The listing builds one solid part. Answer for the finished solid, in the listing's coordinates (mm). A direction names the side the tool comes from. Round coordinates to 2 decimals unless told otherwise and drop trailing zeros. Write each loop counter-clockwise with the first axis right and the second up, starting at its lowest first coordinate (ties: lowest second). Pieces come first, ordered by that corner, then holes. Notation, with made-up numbers: (36, 18) - (64, 18) arc R11 cw to (64, 24) - close; hole circle Ø7 at (84.25, 47.5). An arc over 180 degrees is marked (long way). Return JSON: item names as keys, results as strings. Group by question number.
(1) Which of the six approach directions +Z, -Z, +X, -X, +Y, -Y give full straight-line access (tool end or side, diameter ignored) to faces 1 (the cylindrical face through (11.331, 39.567, -36.024)), 2 (the cylindrical face through (15.722, 3.565, 0.423))?
(2) Determine the mould class of faces 3 (the cylindrical face through (-6.834, 2.974, -1.517)), 4 (the cylindrical face through (-11.517, 39.567, 35.956)), 5 (the cylindrical face through (-27.16, 39.57, 41.47)), 6 (the flat face through (7, 42.032, 1)) for opening direction Z: +Z half, -Z half, draft (parallel to the pull), parting line (faces both ways), or undercut.
(3) Section A-A, the plane x = -5 is taken. Give the number of separate pieces and of enclosed holes in the cut face, then the cut area to 3 significant figures.
(4) Section C-C, the plane z = 22 is taken. Write down the section's boundary in (x, y).
(5) Find the intervals of material crossed by line 1 along X through (y, z) = (3, 0) (3 decimals); line 2 along Y through (x, z) = (6, 14); line 3 along X through (y, z) = (6.5, 0) (3 decimals), in increasing order. Write a range as [from, to].
(6) Each of these flat-tipped pins is pushed along its axis until it touches: pin 1 (6 mm diameter, centred on x = -15, y = 34, fed in from +Z); pin 2 (3.5 mm diameter, centred on x = -6.096, z = 38.1, fed in from +Y); pin 3 (1 mm diameter, centred on y = 37, z = 30, fed in from -X); pin 4 (17 mm diameter, centred on x = 0, z = 0, fed in from +Y). Where does it stop, or does it pass through?
(7) Section D-D, the plane y = 19.5 is taken. Write down the section's boundary in (x, z) (3 decimals), then the cut area to 3 significant figures.
(8) Section B-B, the plane z = -12.5 is taken. Write down the section's boundary in (x, y).
```python
from build123d import *

# Parameters (mm, degrees)
SKETCH1_R                      = 34.925
SKETCH1_R_2                    = 7
BOSS_EXTRUDE1_DEPTH            = 7.032
SKETCH2_R                      = 7.5
CUT_EXTRUDE1_DEPTH             = 1
BOSS_EXTRUDE2_DEPTH            = 30
CUT_EXTRUDE2_DEPTH             = 58.78850448
SKETCH6_R                      = 34.925
SKETCH6_R_2                    = 6.6
BOSS_EXTRUDE6_DEPTH            = 5
CBORE_FOR_M3_SHCS1_D           = 3.3
CBORE_FOR_M3_SHCS1_DEPTH       = 5
CBORE_FOR_M3_SHCS1_CBORE_D     = 6.5
CBORE_FOR_M3_SHCS1_CBORE_DEPTH = 3
SKETCH9_R                      = 3.25
CUT_EXTRUDE3_DEPTH             = 62.732327625
SKETCH10_R                     = 2.2479
BOSS_EXTRUDE7_DEPTH            = 5


with BuildPart() as part:
    # Sketch1 → Boss-Extrude1 (new body)
    with BuildSketch(Plane(origin=(0, 0, 0), x_dir=(1, 0, 0), z_dir=(0, 1, 0))):
        with Locations(Location((0, 0, 0), (0, 0, 270))):
            Circle(SKETCH1_R)
        with Locations(Location((0, 0, 0), (0, 0, 270))):
            Circle(SKETCH1_R_2, mode=Mode.SUBTRACT)
    extrude(amount=BOSS_EXTRUDE1_DEPTH)

    # Sketch2 → Cut-Extrude1 (cut)
    with BuildSketch(Plane(origin=(0, 7.032, 0), x_dir=(1, 0, 0), z_dir=(0, 1, 0))):
        with Locations(Location((0, 0, 0), (0, 0, 270))):
            Circle(SKETCH2_R)
    extrude(amount=-CUT_EXTRUDE1_DEPTH, mode=Mode.SUBTRACT)

    # Sketch3 → Boss-Extrude2 (add)
    with BuildSketch(Plane(origin=(0, 7.032, 0), x_dir=(1, 0, 0), z_dir=(0, 1, 0))):
        with BuildLine():
            Line((19.05, 25.4), (19.05, 29.272053652))
            ThreePointArc((19.05, 29.272053652), (-34.925, 0), (19.05, -29.272053652))
            Line((19.05, -29.272053652), (19.05, -25.4))
            Line((19.05, -25.4), (13.090860361, -25.4))
            ThreePointArc((13.090860361, -25.4), (-28.575, 0), (13.090860361, 25.4))
            Line((13.090860361, 25.4), (19.05, 25.4))
        make_face()
    extrude(amount=BOSS_EXTRUDE2_DEPTH)

    # Sketch3<3> → Cut-Extrude2 (cut, through all)
    with BuildSketch(Plane(origin=(0, 7.032, 0), x_dir=(1, 0, 0), z_dir=(0, 1, 0))):
        with BuildLine():
            ThreePointArc((19.05, -29.272053652), (34.925, 0), (19.05, 29.272053652))
            Line((19.05, 29.272053652), (19.05, 25.4))
            Line((19.05, 25.4), (19.05, -25.4))
            Line((19.05, -25.4), (19.05, -29.272053652))
        make_face()
    extrude(amount=-CUT_EXTRUDE2_DEPTH, mode=Mode.SUBTRACT)

    # Sketch6 → Boss-Extrude6 (add)
    with BuildSketch(Plane(origin=(0, 37.032, 0), x_dir=(1, 0, 0), z_dir=(0, 1, 0))):
        with Locations(Location((0, 0, 0), (0, 0, 56.944268849))):
            Circle(SKETCH6_R)
        with Locations(Location((0, 0, 0), (0, 0, 270))):
            Circle(SKETCH6_R_2, mode=Mode.SUBTRACT)
    extrude(amount=BOSS_EXTRUDE6_DEPTH)

    # CBORE for M3 SHCS1
    with Locations(Plane(origin=(0, 37.032, 0), x_dir=(-1, 0, 0), z_dir=(0, -1, 0))):
        with Locations((-12.5, 0), (0, -12.5), (0, 12.5), (12.5, 0)):
            CounterBoreHole(CBORE_FOR_M3_SHCS1_D / 2, CBORE_FOR_M3_SHCS1_CBORE_D / 2, CBORE_FOR_M3_SHCS1_CBORE_DEPTH, depth=CBORE_FOR_M3_SHCS1_DEPTH)

    # Sketch9 → Cut-Extrude3 (cut, through all)
    with BuildSketch(Plane.XZ.offset(-37.032)):
        with Locations(Location((0, 12.5, 0), (0, 0, 270))):
            Circle(SKETCH9_R)
        with Locations(Location((12.5, 0, 0), (0, 0, 270))):
            Circle(SKETCH9_R)
        with Locations(Location((0, -12.5, 0), (0, 0, 270))):
            Circle(SKETCH9_R)
        with Locations(Location((-12.5, 0, 0), (0, 0, 270))):
            Circle(SKETCH9_R)
    extrude(amount=CUT_EXTRUDE3_DEPTH, mode=Mode.SUBTRACT)

    # Sketch10 → Boss-Extrude7 (add)
    with BuildSketch(Plane(origin=(0, 42.032, 0), x_dir=(1, 0, 0), z_dir=(0, 1, 0))):
        with BuildLine():
            Line((-28.684888393, 38.84902648), (-34.407107147, 5.992211842))
            Line((-34.407107147, 5.992211842), (0, 34.925))
            Line((0, 34.925), (34.407107147, 5.992211842))
            Line((34.407107147, 5.992211842), (28.684888393, 38.84902648))
            ThreePointArc((28.684888393, 38.84902648), (27.193689744, 41.44130591), (24.384, 42.465625))
            Line((24.384, 42.465625), (-24.384, 42.465625))
            ThreePointArc((-24.384, 42.465625), (-27.193689744, 41.44130591), (-28.684888393, 38.84902648))
        make_face()
        with Locations(Location((-24.384, 38.1, 0), (0, 0, 270))):
            Circle(SKETCH10_R, mode=Mode.SUBTRACT)
        with Locations(Location((-18.288, 38.1, 0), (0, 0, 270))):
            Circle(SKETCH10_R, mode=Mode.SUBTRACT)
        with Locations(Location((-12.192, 38.1, 0), (0, 0, 270))):
            Circle(SKETCH10_R, mode=Mode.SUBTRACT)
        with Locations(Location((-6.096, 38.1, 0), (0, 0, 270))):
            Circle(SKETCH10_R, mode=Mode.SUBTRACT)
        with Locations(Location((0, 38.1, 0), (0, 0, 270))):
            Circle(SKETCH10_R, mode=Mode.SUBTRACT)
        with Locations(Location((6.096, 38.1, 0), (0, 0, 270))):
            Circle(SKETCH10_R, mode=Mode.SUBTRACT)
        with Locations(Location((12.192, 38.1, 0), (0, 0, 270))):
            Circle(SKETCH10_R, mode=Mode.SUBTRACT)
        with Locations(Location((18.288, 38.1, 0), (0, 0, 270))):
            Circle(SKETCH10_R, mode=Mode.SUBTRACT)
        with Locations(Location((24.384, 38.1, 0), (0, 0, 270))):
            Circle(SKETCH10_R, mode=Mode.SUBTRACT)
    boss_extrude7 = extrude(amount=-BOSS_EXTRUDE7_DEPTH)

    # Mirror1: Boss-Extrude7 across plane
    add(boss_extrude7.mirror(Plane.XY))


solid = part.part
```
Working result:
{
 "1": {"face 1": "+Y, -Y", "face 2": "-Y"},
 "2": {"face 3": "undercut", "face 4": "undercut", "face 5": "+Z half", "face 6": "draft"},
 "3": {"separate pieces": "4", "enclosed holes": "0", "area": "1,140 mm^2"},
 "4": {"outline": "(-31.62, 37.03) - (-27.12, 37.03) - (-27.12, 0) - (19.05, 0) - (19.05, 7.03) - (-18.24, 7.03) - (-18.24, 37.03) - (31.62, 37.03) - (31.62, 42.03) - (-31.62, 42.03) - close"},
 "5": {"line 1": "x = [-34.925, -15.75], [-9.25, -7], [7, 9.25], [15.75, 19.05]", "line 2": "y = [0, 7.03], [37.03, 42.03]", "line 3": "x = [-34.925, -15.75], [-9.25, -7.5], [7.5, 9.25], [15.75, 19.05]"},
 "6": {"pin 1": "stops at z = 32.8", "pin 2": "passes through", "pin 3": "stops at x = -30.31", "pin 4": "stops at y = 42.03"},
 "7": {"outline": "(13.091, -25.4) arc R28.575 cw (long way) to (13.091, 25.4) - (19.05, 25.4) - (19.05, 29.272) arc R34.925 ccw (long way) to (19.05, -29.272) - (19.05, -25.4) - close", "area": "871 mm^2"},
 "8": {"outline": "(-33.27, 37.03) - (-32.61, 37.03) - (-32.61, 0) - (-3.25, 0) - (-3.25, 7.03) - (-25.7, 7.03) - (-25.7, 37.03) - (-3.25, 37.03) - (-3.25, 40.03) - (-1.65, 40.03) - (-1.65, 42.03) - (-33.27, 42.03) - close; (1.65, 40.03) - (3.25, 40.03) - (3.25, 37.03) - (33.27, 37.03) - (33.27, 42.03) - (1.65, 42.03) - close; (3.25, 0) - (19.05, 0) - (19.05, 7.03) - (3.25, 7.03) - close"}
}
